Here's how the part is built. I have some questions about the finished solid (model axes, mm). A direction names the side the tool comes from. Coordinates: 2 decimals unless noted, no trailing zeros. Loops run counter-clockwise (first coordinate to the right, second up) from the corner with the lowest first, then second, coordinate; pieces in that order, holes last. Notation, with made-up numbers: (25, 22.5) -> (78, 22.5) arc R18 ccw to (78, 57.5) -> close; hole circle Ø6 at (13.25, -3.5). An arc over 180 degrees is marked (long way). Use CSV: the item, a comma, the result in double quotes. Start each with the question number.
from build123d import *

# Parameters (mm, degrees)
BOSS_EXTRUDE1_DEPTH = 3
BOSS_EXTRUDE2_DEPTH = 60
SKETCH3_R           = 1.5
CUT_EXTRUDE1_DEPTH  = 30
CUT_EXTRUDE2_START  = -15
SKETCH3_3_R         = 1.5
CUT_EXTRUDE2_DEPTH  = 5


with BuildPart() as part:
    # Sketch1 → Boss-Extrude1 (new body)
    # profile 1 of 2: a face of its own
    with BuildSketch(Plane(origin=(0, 0, 0), x_dir=(0, 1, 0), z_dir=(0, 0, 1))):
        with BuildLine():
            ThreePointArc((-50, 57), (-49.121320344, 59.121320344), (-47, 60))
            Line((-47, 60), (47, 60))
            ThreePointArc((47, 60), (49.121320344, 59.121320344), (50, 57))
            Line((50, 57), (50, -57))
            ThreePointArc((50, -57), (49.121320344, -59.121320344), (47, -60))
            Line((47, -60), (-47, -60))
            ThreePointArc((-47, -60), (-49.121320344, -59.121320344), (-50, -57))
            Line((-50, -57), (-50, 57))
        make_face()
        with BuildLine():
            Line((-47, 47), (-47, -47))
            ThreePointArc((-47, -47), (-44.071067812, -54.071067812), (-37, -57))
            Line((-37, -57), (37, -57))
            ThreePointArc((37, -57), (44.071067812, -54.071067812), (47, -47))
            Line((47, -47), (47, 47))
            ThreePointArc((47, 47), (44.071067812, 54.071067812), (37, 57))
            Line((37, 57), (-37, 57))
            ThreePointArc((-37, 57), (-44.071067812, 54.071067812), (-47, 47))
        make_face(mode=Mode.SUBTRACT)
    # profile 2 of 2: a face of its own
    with BuildSketch(Plane(origin=(0, 0, 0), x_dir=(0, 1, 0), z_dir=(0, 0, 1))):
        with BuildLine():
            ThreePointArc((-47, 47), (-44.071067812, 54.071067812), (-37, 57))
            Line((-37, 57), (37, 57))
            ThreePointArc((37, 57), (44.071067812, 54.071067812), (47, 47))
            Line((47, 47), (47, -47))
            ThreePointArc((47, -47), (44.071067812, -54.071067812), (37, -57))
            Line((37, -57), (-37, -57))
            ThreePointArc((-37, -57), (-44.071067812, -54.071067812), (-47, -47))
            Line((-47, -47), (-47, 47))
        make_face()
    extrude(amount=BOSS_EXTRUDE1_DEPTH)

    # Sketch1_3 → Boss-Extrude2 (add)
    with BuildSketch(Plane(origin=(0, 0, 0), x_dir=(0, 1, 0), z_dir=(0, 0, 1))):
        with BuildLine():
            ThreePointArc((-50, 57), (-49.121320344, 59.121320344), (-47, 60))
            Line((-47, 60), (47, 60))
            ThreePointArc((47, 60), (49.121320344, 59.121320344), (50, 57))
            Line((50, 57), (50, -57))
            ThreePointArc((50, -57), (49.121320344, -59.121320344), (47, -60))
            Line((47, -60), (-47, -60))
            ThreePointArc((-47, -60), (-49.121320344, -59.121320344), (-50, -57))
            Line((-50, -57), (-50, 57))
        make_face()
        with BuildLine():
            Line((-47, 47), (-47, -47))
            ThreePointArc((-47, -47), (-44.071067812, -54.071067812), (-37, -57))
            Line((-37, -57), (37, -57))
            ThreePointArc((37, -57), (44.071067812, -54.071067812), (47, -47))
            Line((47, -47), (47, 47))
            ThreePointArc((47, 47), (44.071067812, 54.071067812), (37, 57))
            Line((37, 57), (-37, 57))
            ThreePointArc((-37, 57), (-44.071067812, 54.071067812), (-47, 47))
        make_face(mode=Mode.SUBTRACT)
    extrude(amount=BOSS_EXTRUDE2_DEPTH)

    # Sketch3 → Cut-Extrude1 (cut)
    with BuildSketch(Plane.XY.offset(60)):
        with Locations((-56, 46)):
            Circle(SKETCH3_R)
        with Locations((56, 46)):
            Circle(SKETCH3_R)
        with Locations((56, -46)):
            Circle(SKETCH3_R)
        with Locations((-56, -46)):
            Circle(SKETCH3_R)
    extrude(amount=-CUT_EXTRUDE1_DEPTH, mode=Mode.SUBTRACT)

    # Sketch3_3 → Cut-Extrude2 (cut)
    # profile 1 of 4: a face of its own
    with BuildSketch(Plane.XY.offset(60).offset(CUT_EXTRUDE2_START)):
        with BuildLine():
            Line((-53, 45), (-53, 47.732050808))
            Line((-53, 47.732050808), (-56, 49.464101615))
            Line((-56, 49.464101615), (-59, 47.732050808))
            Line((-59, 47.732050808), (-59, 44.267949192))
            Line((-59, 44.267949192), (-56, 42.535898385))
            Line((-56, 42.535898385), (-54.842890525, 43.203955852))
            ThreePointArc((-54.842890525, 43.203955852), (-53.979459017, 44.161504858), (-53, 45))
        make_face()
        with Locations((-56, 46)):
            Circle(SKETCH3_3_R, mode=Mode.SUBTRACT)
    # profile 2 of 4: a face of its own
    with BuildSketch(Plane.XY.offset(60).offset(CUT_EXTRUDE2_START)):
        with BuildLine():
            Line((59, 47.732050808), (56, 49.464101615))
            Line((56, 49.464101615), (53, 47.732050808))
            Line((53, 47.732050808), (53, 45))
            ThreePointArc((53, 45), (53.979459017, 44.161504858), (54.842890525, 43.203955852))
            Line((54.842890525, 43.203955852), (56, 42.535898385))
            Line((56, 42.535898385), (59, 44.267949192))
            Line((59, 44.267949192), (59, 47.732050808))
        make_face()
        with Locations((56, 46)):
            Circle(SKETCH3_3_R, mode=Mode.SUBTRACT)
    # profile 3 of 4: a face of its own
    with BuildSketch(Plane.XY.offset(60).offset(CUT_EXTRUDE2_START)):
        with BuildLine():
            Line((59, -44.267949192), (56, -42.535898385))
            Line((56, -42.535898385), (54.842890525, -43.203955852))
            ThreePointArc((54.842890525, -43.203955852), (53.979459017, -44.161504858), (53, -45))
            Line((53, -45), (53, -47.732050808))
            Line((53, -47.732050808), (56, -49.464101615))
            Line((56, -49.464101615), (59, -47.732050808))
            Line((59, -47.732050808), (59, -44.267949192))
        make_face()
        with Locations((56, -46)):
            Circle(SKETCH3_3_R, mode=Mode.SUBTRACT)
    # profile 4 of 4: a face of its own
    with BuildSketch(Plane.XY.offset(60).offset(CUT_EXTRUDE2_START)):
        with BuildLine():
            Line((-54.842890525, -43.203955852), (-56, -42.535898385))
            Line((-56, -42.535898385), (-59, -44.267949192))
            Line((-59, -44.267949192), (-59, -47.732050808))
            Line((-59, -47.732050808), (-56, -49.464101615))
            Line((-56, -49.464101615), (-53, -47.732050808))
            Line((-53, -47.732050808), (-53, -45))
            ThreePointArc((-53, -45), (-53.979459017, -44.161504858), (-54.842890525, -43.203955852))
        make_face()
        with Locations((-56, -46)):
            Circle(SKETCH3_3_R, mode=Mode.SUBTRACT)
    extrude(amount=-CUT_EXTRUDE2_DEPTH, mode=Mode.SUBTRACT)


solid = part.part
1) For P1, Ø2, axis at x = -8, y = 34, coming from the +Z side; P2, Ø0.9, axis at x = 55.5, y = 45.5, coming from the +Z side, each with a flat end and sliding along its axis, tell me the tip position at first contact or that it passes through.
2) I want a section at D-D, the plane x = 26. Please give me the cut outline in (y, z), plus the area to 3 significant figures.
3) Please list where these lines run through material, in increasing order: L1, parallel to Y at x = -32, z = 15; L2, parallel to X at y = 33.5, z = 5; L3, parallel to Y at x = -56, z = 36. Write a range as [from, to].
4) I want a section at B-B, the plane y = -28.5. Please give me the cut outline in (x, z).
5) I want a section at C-C, the plane z = 14. Please give me the cut outline in (x, y), plus the area to 3 significant figures.
6) Which directions (+Z, -Z, +X, -X, +Y, -Y) give clear straight access to the entire face, cutting with the end or side of a thin tool? Please do faces 4 (the face through (-56, -46, 30)), 5 (the face through (-53, -46, 43)), 6 (the face through (1, -50, 30)).
7) I want a section at A-A, the plane z = 37. Please give me the cut outline in (x, y).
8) Thinking about a two-plate mould opening in Z: for faces 1 (the face through (53, 46, 43)), 2 (the face through (-1, 1, 3)), 3 (the face through (-1, 1, 0)), which applies, pulls with the +Z half, pulls with the -Z half, needs draft (parallel to the pull), parting line crosses it, or undercut?
Return value:
1,P1,"stops at z = 3"
1,P2,"stops at z = 30"
2,outline,"(-50, 0) -> (50, 0) -> (50, 60) -> (47, 60) -> (47, 3) -> (-47, 3) -> (-47, 60) -> (-50, 60) -> close"
2,area,"642 mm²"
3,L1,"y = [-50, -47], [47, 50]"
3,L2,"x = [-60, -57], [57, 60]"
3,L3,"y = [-50, -47.5], [-44.5, -41.36], [41.36, 44.5], [47.5, 50]"
4,outline,"(-60, 0) -> (60, 0) -> (60, 60) -> (57, 60) -> (57, 3) -> (-57, 3) -> (-57, 60) -> (-60, 60) -> close"
5,outline,"(-60, -47) arc R3 ccw to (-57, -50) -> (57, -50) arc R3 ccw to (60, -47) -> (60, 47) arc R3 ccw to (57, 50) -> (-57, 50) arc R3 ccw to (-60, 47) -> close; hole (-57, -37) arc R10 ccw to (-47, -47) -> (47, -47) arc R10 ccw to (57, -37) -> (57, 37) arc R10 ccw to (47, 47) -> (-47, 47) arc R10 ccw to (-57, 37) -> close"
5,area,"1,360 mm²"
6,face 4,"+Z"
6,face 5,"none"
6,face 6,"+Z, -Z, +X, -X, -Y"
7,outline,"(-60, -47) arc R3 ccw to (-57, -50) -> (57, -50) arc R3 ccw to (60, -47) -> (60, 47) arc R3 ccw to (57, 50) -> (-57, 50) arc R3 ccw to (-60, 47) -> close; hole circle Ø3 at (-56, -46); hole circle Ø3 at (-56, 46); hole (-57, -37) arc R10 ccw to (-47, -47) -> (47, -47) arc R10 ccw to (57, -37) -> (57, 37) arc R10 ccw to (47, 47) -> (-47, 47) arc R10 ccw to (-57, 37) -> close; hole circle Ø3 at (56, -46); hole circle Ø3 at (56, 46)"
8,face 1,"undercut"
8,face 2,"pulls with the +Z half"
8,face 3,"pulls with the -Z half"
